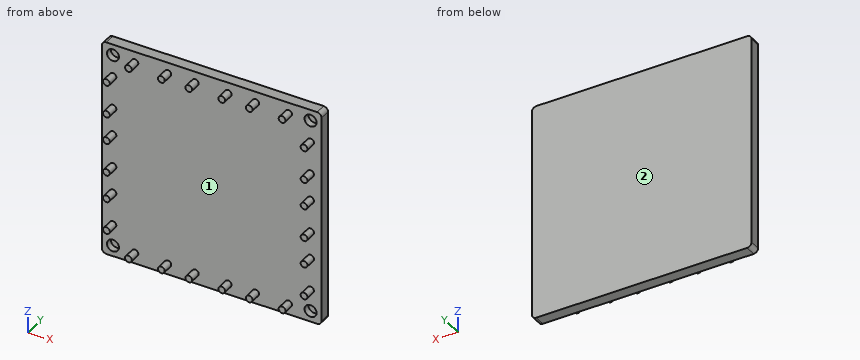
Autodesk Inventor part; units mm, degrees
ref_plane "YZ Plane" through (0, 0, 0) normal (1, 0, 0) x (0, 1, 0)
ref_plane "XZ Plane" through (0, 0, 0) normal (0, 1, 0) x (-1, 0, 0)
ref_plane "XY Plane" through (0, 0, 0) normal (0, 0, 1) x (1, 0, 0)
sketch "Esquisse1" plane through (0, 0, 0) normal (0, 1, 0) x (-1, 0, 0)
  line L0 (0, 0) -> (100, 0)
  line L1 (100, 0) -> (100, -100)
  line L2 (100, -100) -> (0, -100)
  line L3 (0, -100) -> (0, 0)
  dimension "d0" = 100
  dimension "d1" = 100
extrude "Extrusion1" add sketch "Esquisse1" along normal blind 5
sketch "Esquisse3" plane through (0, 0, 0) normal (0, -1, 0) x (1, 0, 0)
  line L0 (0, -100) -> (-100, -100)
  line L1 (0, -100) -> (-4.9999, -95)
  circle A0 centre (-4.9999, -95) radius 1.6952
  point P0 (0, 0)
  dimension "d4" = 7.071
hole "Perçage1" at (-4.9999, 0, -95) direction (0, 1, 0) diameter 5.5 depth 3
pattern_linear "Réseau rectangulaire1" count 2 spacing 90 along (0, 0, 1) count 2 spacing 90 along (-1, 0, 0) of "Perçage1"
fillet "Congé1" radius 2 4 edges at (0, 2.5, 0) (-100, 2.5, 0) (-100, 2.5, -100) (0, 2.5, -100)
sketch "Esquisse7" plane through (0, 0, 0) normal (0, -1, 0) x (1, 0, 0)
  circle A0 centre (-4.9999, -5) radius 2.4794
  circle A1 centre (-94.9999, -95) radius 2.4794
  line L0 (-4.9999, -5) -> (-94.9999, -5)
  line L1 (-94.9999, -5) -> (-94.9999, -95)
  line L2 (-94.9999, -95) -> (-4.9999, -95)
  line L3 (-4.9999, -95) -> (-4.9999, -5)
  line L4 (-49.9999, -5) -> (-49.9999, -95)
  line L5 (-4.9999, -50) -> (-94.9999, -50)
  line L6 (-49.9999, -95) -> (-42.4999, -95)
  line L7 (-49.9999, -95) -> (-57.4999, -95)
  circle A2 centre (-57.4999, -95) radius 1.55
  circle A3 centre (-42.4999, -95) radius 1.55
  line L8 (-94.9999, -95) -> (-84.9999, -95)
  line L9 (-84.9999, -95) -> (-69.9999, -95)
  circle A4 centre (-69.9999, -95) radius 1.55
  circle A5 centre (-84.9999, -95) radius 1.55
  circle A6 centre (-4.9999, -95) radius 2.4794
  line L10 (-4.9999, -95) -> (-14.9999, -95)
  line L11 (-14.9999, -95) -> (-29.9999, -95)
  circle A7 centre (-14.9999, -95) radius 1.55
  circle A8 centre (-29.9999, -95) radius 1.55
  circle A9 centre (-14.9999, -5) radius 1.55
  circle A10 centre (-29.9999, -5) radius 1.55
  circle A11 centre (-42.4999, -5) radius 1.55
  circle A12 centre (-57.4999, -5) radius 1.55
  circle A13 centre (-69.9999, -5) radius 1.55
  circle A14 centre (-84.9999, -5) radius 1.55
  circle A15 centre (-4.9999, -85) radius 1.55
  circle A16 centre (-4.9999, -70) radius 1.55
  circle A17 centre (-4.9999, -57.5) radius 1.55
  circle A18 centre (-4.9999, -42.5) radius 1.55
  circle A19 centre (-4.9999, -30) radius 1.55
  circle A20 centre (-4.9999, -15) radius 1.55
  circle A21 centre (-94.9999, -15) radius 1.55
  circle A22 centre (-94.9999, -30) radius 1.55
  circle A23 centre (-94.9999, -42.5) radius 1.55
  circle A24 centre (-94.9999, -57.5) radius 1.55
  circle A25 centre (-94.9999, -70) radius 1.55
  circle A26 centre (-94.9999, -85) radius 1.55
  point P0 (0, 0)
  dimension "d35" = 7.5
  dimension "d36" = 7.5
  dimension "d37" = 3.1
  dimension "d38" = 3.1
  dimension "d39" = 10
  dimension "d40" = 15
  dimension "d41" = 3.1
  dimension "d42" = 3.1
  dimension "d43" = 10
  dimension "d44" = 15
  dimension "d45" = 3.1
  dimension "d46" = 3.1
  dimension "d49" = 90
  dimension "d56" = 270
  dimension "d60" = 90
extrude "Extrusion3" add sketch "Esquisse7" along normal blind 5 contours A9 L0 | L0 A9 | A20 L3 | L3 A20 | A10 L0 | L0 A10 | A19 L3 | L3 A19 | A11 L0 | L0 A11 | A18 L3 | L3 A18 | A12 L0 | L0 A12 | A17 L3 | L3 A17 | A13 L0 | L0 A13 | A2 L2 | L2 A2 | A3 L2 | L2 A3 | A23 L1 | L1 A23 | A24 L1 | L1 A24 | A16 L3 | L3 A16 | A14 L0 | L0 A14 | A4 L2 | L2 A4 | A8 L2 | L2 A8 | A22 L1 | L1 A22 | A25 L1 | L1 A25 | A15 L3 | L3 A15 | A5 L2 | L2 A5 | A7 L2 | L2 A7 | A21 L1 | L1 A21 | A26 L1 | L1 A26
thread "Filetage1"
thread "Filetage2"
thread "Filetage3"
thread "Filetage4"
thread "Filetage5"
thread "Filetage6"
thread "Filetage7"
thread "Filetage8"
thread "Filetage9"
thread "Filetage10"
thread "Filetage11"
thread "Filetage12"
thread "Filetage13"
thread "Filetage14"
thread "Filetage15"
thread "Filetage16"
thread "Filetage17"
thread "Filetage18"
thread "Filetage19"
thread "Filetage20"
thread "Filetage21"
thread "Filetage22"
thread "Filetage23"
thread "Filetage24"
properties part number "plateau"
Read the model definition and answer for the solid it produces. Units are mm, in the model's axes. Face numbers are marked on the shaded views. Give positions to 0.01 mm unless a question says otherwise; leave off trailing zeros. Loops run counter-clockwise (first coordinate to the right, second up) from the corner with the lowest first, then second, coordinate; pieces in that order, holes last.
Item 1: Each of these flat-tipped pins is pushed along its axis until it touches: pin 1 Ø6.5 at (x, z) = (-95, -5) entering from -Y; pin 2 Ø1.6 at (x, z) = (-95, -93.5) entering from -Y. Where does it stop, or does it pass through?
Item 2: The part is cut by section B-B (x = -36). Write down the section's boundary in (y, z).
Item 3: Find the intervals of material crossed by line 1 along X through (y, z) = (2.1, -95); line 2 along Y through (x, z) = (-87.5, -17.5), in increasing order.
Item 4: The mould has two halves that part along Z. Classify the marked faces 1 and 2: released by +Z, released by -Z, zero draft, split by the parting line, or undercut.
Item 5: The part is cut by section A-A (z = -57.5). Write down the section's boundary in (x, y).
Taken from the geometry:
1. pin 1: stops at y = 0
1. pin 2: stops at y = 3
2. outline: (0, -100) - (5, -100) - (5, 0) - (0, 0) - close
3. line 1: x = -100 to -97.75, -92.25 to -7.75, -2.25 to 0
3. line 2: y = 0 to 5
4. face 1: undercut
4. face 2: zero draft
5. outline: (-100, 0) - (-96.55, 0) - (-96.55, -5) - (-93.45, -5) - (-93.45, 0) - (-6.55, 0) - (-6.55, -5) - (-3.45, -5) - (-3.45, 0) - (0, 0) - (0, 5) - (-100, 5) - close
